Geometry check sheet. Reference: the model listing, model coordinates, mm. A direction names the side the tool comes from. Round coordinates to 2 decimals unless told otherwise and drop trailing zeros. Write each loop counter-clockwise with the first axis right and the second up, starting at its lowest first coordinate (ties: lowest second). Pieces come first, ordered by that corner, then holes. Notation, with made-up numbers: (-4, -37.75) - (7, -37.75) arc R34 ccw to (7, -7.75) - close; hole circle Ø9 at (-4, -32.75). An arc over 180 degrees is marked (long way). Return JSON: item names as keys, results as strings.
```python
from build123d import *

# Parameters (mm, degrees)
SKETCH046_R     = 7.3025
SKETCH046_R_2   = 3.7465
PAD007_DEPTH    = 0.762
POCKET006_DEPTH = 0.763
FILLET004_R     = 0.79375
FILLET005_R     = 0.635


with BuildPart() as part:
    # Sketch046 → Pad007 (new body)
    with BuildSketch(Plane.XZ):
        Circle(SKETCH046_R)
        Circle(SKETCH046_R_2, mode=Mode.SUBTRACT)
    extrude(amount=PAD007_DEPTH)

    # Sketch047 (on Face4 of Pad007) → Pocket006 (cut, through all)
    with BuildSketch(Plane.XZ.offset(0.762)):
        with BuildLine():
            Line((-4.545908, -5.715), (-3.087808, -2.121721))
            Line((-3.087808, -2.121721), (-2.896797, -1.651))
            Line((-2.896797, -1.651), (-3.415378, -1.539953))
            Line((-3.415378, -1.539953), (-5.614107, -1.069124))
            ThreePointArc((-1.531348, 5.506015), (-4.855151, 3.014752), (-5.614107, -1.069124))
            Line((-0.291377, 3.735152), (-1.531348, 5.506015))
            Line((-0.291377, 3.735152), (0, 3.319023))
            Line((0, 3.319023), (0.291377, 3.735152))
            Line((0.291377, 3.735152), (1.531348, 5.506015))
            ThreePointArc((5.614107, -1.069124), (4.855151, 3.014752), (1.531348, 5.506015))
            Line((3.415378, -1.539953), (5.614107, -1.069124))
            Line((3.415378, -1.539953), (2.896797, -1.651))
            Line((2.896797, -1.651), (3.087808, -2.121721))
            Line((4.545908, -5.715), (3.087808, -2.121721))
            Line((4.545908, -5.715), (5.040156, -5.715))
            ThreePointArc((-5.040156, -5.715), (0, -7.62), (5.040156, -5.715))
            Line((-4.545908, -5.715), (-5.040156, -5.715))
        make_face()
    extrude(amount=-POCKET006_DEPTH, mode=Mode.SUBTRACT)

    # Fillet004
    fillet004_edges = [part.edges().sort_by_distance(p)[0] for p in [
        (-4.545908, -0.381, -5.715),
        (4.545908, -0.381, -5.715),
    ]]
    fillet(fillet004_edges, radius=FILLET004_R)

    # Fillet005
    fillet005_edges = [part.edges().sort_by_distance(p)[0] for p in [
        (-5.614107, -0.381, -1.069124),
        (5.614107, -0.381, -1.069124),
        (-1.531348, -0.381, 5.506015),
        (1.531348, -0.381, 5.506015),
    ]]
    fillet(fillet005_edges, radius=FILLET005_R)


with BuildPart() as part_1:
    # Body005 placement: moved
    add(part.part.moved(Location((0, 45.2755, 0))))


solid = part_1.part
```
(1) Section check A-A, the plane z = 0. Enter the section's corners in (x, y) (1 decimal).
Response values:
{"outline": "(-7.3, 44.5) - (-5.7, 44.5) - (-5.7, 45.3) - (-7.3, 45.3) - close; (5.7, 44.5) - (7.3, 44.5) - (7.3, 45.3) - (5.7, 45.3) - close"}
(2) Section check D-D, the plane x = 0. Enter the section's corners in (y, z).
Response values:
{"outline": "(44.51, 3.75) - (45.28, 3.75) - (45.28, 7.3) - (44.51, 7.3) - close"}
(3) Section check C-C, the plane y = 44.85. Enter the section's corners in (x, z) (1 decimal), plus the area to 3 significant figures.
Response values:
{"outline": "(-5.7, -0.6) arc R5.7 cw to (-2, 5.4) arc R0.6 cw to (-1.3, 5.1) - (-0.3, 3.7) arc R3.7 cw to (0.3, 3.7) - (1.3, 5.1) arc R0.6 cw to (2, 5.4) arc R5.7 cw to (5.7, -0.6) arc R0.6 cw to (5.2, -1.2) - (3.4, -1.5) arc R3.7 cw to (3.1, -2.1) - (4.1, -4.6) arc R0.8 ccw to (5.4, -4.9) arc R7.3 ccw (long way) to (-5.4, -4.9) arc R0.8 ccw to (-4.1, -4.6) - (-3.1, -2.1) arc R3.7 cw to (-3.4, -1.5) - (-5.2, -1.2) arc R0.6 cw to start", "area": "61.9 mm^2"}
(4) Release check for a two-part mould opening along X. For faces 1 (the face through (0.2, 44.9, 7.3)), 2 (the face through (-0.77, 44.89, 4.42)), 3 (the face through (0, 45.276, 5)) record: pulls with the +X half, pulls with the -X half, needs draft (parallel to the pull), parting line crosses it, or undercut.
Response values:
{"face 1": "parting line crosses it", "face 2": "undercut", "face 3": "needs draft"}
(5) Gauge pin test, flat end, axial feed: pin 1 (1 mm diameter, centred on x = -1.5, z = 2, fed in from +Y). Record the tip position at first contact, or that the pin passes through.
Response values:
{"pin 1": "passes through"}
(6) Material ranges on line 1 along X through (y, z) = (44.9, 0) (1 decimal); line 2 along X through (y, z) = (45.15, 4); line 3 along X through (y, z) = (44.95, -3.75), recorded low to high. Write a range as [from, to].
Response values:
{"line 1": "x = [-7.3, -5.7], [5.7, 7.3]", "line 2": "x = [-6.11, -4.08], [-0.48, 0.48], [4.08, 6.11]", "line 3": "x = [-6.27, -3.75], [3.75, 6.27]"}
(7) Section check B-B, the plane x = -3.75. Enter the section's corners in (y, z).
Response values:
{"outline": "(44.51, -3.75) - (45.28, -3.75) - (45.28, -1.47) - (44.51, -1.47) - close; (44.51, 4.31) - (45.28, 4.31) - (45.28, 6.27) - (44.51, 6.27) - close"}
(8) Access from +Z, -Z, +X, -X, +Y, -Y to the whole of each face (thin tool, end or side, straight path). Record for faces 4 (the face through (0, 44.514, 5)), 5 (the face through (3.607, 44.889, -3.4)), 6 (the face through (-4.836, 44.889, 3.046)).
Response values:
{"face 4": "+Z, -Z, +X, -X, -Y", "face 5": "-Z, +Y, -Y", "face 6": "+Y, -Y"}
